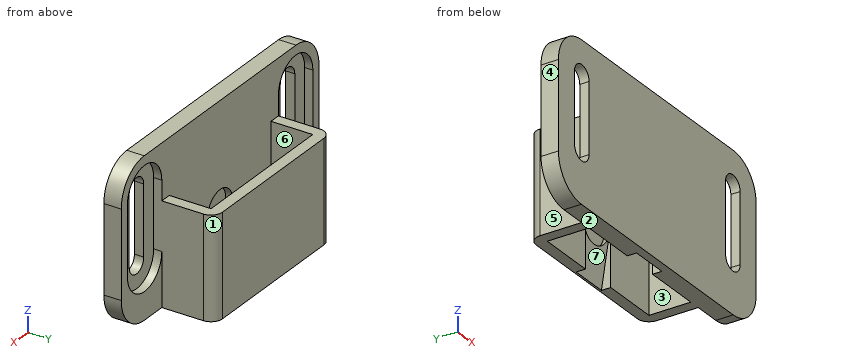
```python
from build123d import *

# Parameters (mm, degrees)
BOSS_EXTRUDE1_DEPTH = 3
CUT_EXTRUDE1_DEPTH  = 1.4
CUT_EXTRUDE2_DEPTH  = 3
BOSS_EXTRUDE2_DEPTH = 17.5
FILLET1_R           = 2
SKETCH8_R           = 3.3
CUT_EXTRUDE3_DEPTH  = 1.2
CUT_EXTRUDE4_START  = -1.2
SKETCH9_R           = 3.3
CUT_EXTRUDE4_DEPTH  = 1.2


with BuildPart() as part:
    # Sketch1 → Boss-Extrude1 (new body)
    with BuildSketch(Plane(origin=(0, 0, 0), x_dir=(1, 0, 0), z_dir=(0, 1, 0))):
        with BuildLine():
            Line((-19.85, -13.5), (19.85, -13.5))
            ThreePointArc((19.85, -13.5), (24.092640687, -11.742640687), (25.85, -7.5))
            Line((25.85, -7.5), (25.85, 7.5))
            ThreePointArc((25.85, 7.5), (24.092640687, 11.742640687), (19.85, 13.5))
            Line((19.85, 13.5), (-19.85, 13.5))
            ThreePointArc((-19.85, 13.5), (-24.092640687, 11.742640687), (-25.85, 7.5))
            Line((-25.85, 7.5), (-25.85, -7.5))
            ThreePointArc((-25.85, -7.5), (-24.092640687, -11.742640687), (-19.85, -13.5))
        make_face()
    extrude(amount=BOSS_EXTRUDE1_DEPTH)

    # Sketch2 → Cut-Extrude1 (cut)
    with BuildSketch(Plane(origin=(0, 3, 0), x_dir=(1, 0, 0), z_dir=(0, 1, 0))):
        with BuildLine():
            Line((-24.25, 4.3), (-24.25, -7.4))
            ThreePointArc((-24.25, -7.4), (-19.75, -11.9), (-15.25, -7.4))
            Line((-15.25, -7.4), (-15.25, 4.3))
            ThreePointArc((-15.25, 4.3), (-19.75, 8.8), (-24.25, 4.3))
        make_face()
        with BuildLine():
            Line((24.25, 4.3), (24.25, -7.4))
            ThreePointArc((24.25, -7.4), (19.75, -11.9), (15.25, -7.4))
            Line((15.25, -7.4), (15.25, 4.3))
            ThreePointArc((15.25, 4.3), (19.75, 8.8), (24.25, 4.3))
        make_face()
    extrude(amount=-CUT_EXTRUDE1_DEPTH, mode=Mode.SUBTRACT)

    # Sketch4 → Cut-Extrude2 (cut)
    with BuildSketch(Plane(origin=(0, 3, 0), x_dir=(1, 0, 0), z_dir=(0, 1, 0))):
        with BuildLine():
            Line((-17.85, 4.45), (-17.85, -7.55))
            ThreePointArc((-17.85, -7.55), (-19.75, -9.45), (-21.65, -7.55))
            Line((-21.65, -7.55), (-21.65, 4.45))
            ThreePointArc((-21.65, 4.45), (-19.75, 6.35), (-17.85, 4.45))
        make_face()
        with BuildLine():
            Line((17.85, 4.45), (17.85, -7.55))
            ThreePointArc((17.85, -7.55), (19.75, -9.45), (21.65, -7.55))
            Line((21.65, -7.55), (21.65, 4.45))
            ThreePointArc((21.65, 4.45), (19.75, 6.35), (17.85, 4.45))
        make_face()
    extrude(amount=-CUT_EXTRUDE2_DEPTH, mode=Mode.SUBTRACT)

    # Sketch5 → Boss-Extrude2 (add)
    with BuildSketch(Plane(origin=(0, 0, -13.5), x_dir=(-1, 0, 0), z_dir=(0, 0, -1))):
        Polygon((-13.3, 3), (-13.3, 10.2), (13.3, 10.2), (13.3, 3), (15.25, 3), (15.25, 12.15), (-15.25, 12.15), (-15.25, 3), align=None)
    extrude(amount=-BOSS_EXTRUDE2_DEPTH)

    # Fillet1
    fillet1_edges = [part.edges().sort_by_distance(p)[0] for p in [
        (15.25, 12.15, -4.75),
        (-15.25, 12.15, -4.75),
    ]]
    fillet(fillet1_edges, radius=FILLET1_R)

    # Sketch8 → Cut-Extrude3 (cut)
    with BuildSketch(Plane(origin=(0, 3, 0), x_dir=(1, 0, 0), z_dir=(0, 1, 0))):
        with Locations(Location((0, 4.4, 0), (0, 0, 270))):
            Circle(SKETCH8_R)
    extrude(amount=-CUT_EXTRUDE3_DEPTH, mode=Mode.SUBTRACT)

    # Sketch9 → Cut-Extrude4 (cut)
    with BuildSketch(Plane.XZ.offset(-10.2).offset(CUT_EXTRUDE4_START)):
        with Locations(Location((0, -4.4, 0), (0, 0, 90))):
            Circle(SKETCH9_R)
    extrude(amount=CUT_EXTRUDE4_DEPTH, mode=Mode.SUBTRACT)

    # Sketch11 → Cut-Loft4 section 0
    with BuildSketch(Plane(origin=(0, 0, -13.5), x_dir=(-1, 0, 0), z_dir=(0, 0, -1))):
        with BuildLine():
            Line((-3.3, 11.8), (3.3, 11.8))
            Line((3.3, 11.8), (3.3, 10.2))
            Line((3.3, 10.2), (-3.3, 10.2))
            Line((-3.3, 10.2), (-3.3, 11.8))
        make_face()
    # Sketch12 → Cut-Loft4 section 1
    with BuildSketch(Plane.XY.offset(-4.4)):
        with BuildLine():
            Line((-3.3, 10.2), (3.3, 10.2))
            Line((3.3, 10.2), (3.3, 10.4))
            Line((3.3, 10.4), (-3.3, 10.4))
            Line((-3.3, 10.4), (-3.3, 10.2))
        make_face()
    loft(mode=Mode.SUBTRACT)

    # Sketch11<110> → Cut-Loft7 section 0
    with BuildSketch(Plane(origin=(0, 0, -13.5), x_dir=(-1, 0, 0), z_dir=(0, 0, -1))):
        with BuildLine():
            Line((-3.3, 3), (3.3, 3))
            Line((3.3, 3), (3.3, 1.4))
            Line((3.3, 1.4), (-3.3, 1.4))
            Line((-3.3, 1.4), (-3.3, 3))
        make_face()
    # Sketch12<5> → Cut-Loft7 section 1
    with BuildSketch(Plane.XY.offset(-4.4)):
        with BuildLine():
            Line((-3.3, 3), (3.3, 3))
            Line((3.3, 3), (3.3, 2.8))
            Line((3.3, 2.8), (-3.3, 2.8))
            Line((-3.3, 2.8), (-3.3, 3))
        make_face()
    loft(mode=Mode.SUBTRACT)


solid = part.part
```
Geometry: final body of the model. Coordinates: model frame, mm. Face numbers are marked on the shaded views. A direction names the side the tool comes from. Coordinates: 2 decimals unless noted, no trailing zeros. Order: outer loops, then holes, each group sorted by start corner. A loop starts at its lowest first (then second) coordinate and runs counter-clockwise, first axis right, second up.
Item 1: Section query C-C (x = 14). Output: boundary loops of the cut face in (y, z).
Answer:
outline: (0, -13.5) - (12, -13.5) - (12, 4) - (3, 4) - (3, 13.5) - (0, 13.5) - close
Item 2: Contact query for flat-ended pins moving along their axis: P1, Ø4.5, axis at y = 7.5, z = -2, coming from the -X side; P2, Ø6, axis at x = 19, z = -7, coming from the +Y side; P3, Ø1.5, axis at x = 18, z = -7.5, coming from the +Y side. Output: stop coordinate, or through.
Answer:
P1: stops at x = -15.25
P2: stops at y = 3
P3: stops at y = 1.6
Item 3: Material intervals for line 1 along X through (y, z) = (2, 2); line 2 along X through (y, z) = (2.3, -4.4); line 3 along Y through (x, z) = (-7, 0.75), sorted ascending.
Answer:
line 1: x = -25.85 to -24.25, -15.25 to 15.25, 24.25 to 25.85
line 2: x = -25.85 to -24.25, -15.25 to -3.3, 3.3 to 15.25, 24.25 to 25.85
line 3: y = 0 to 3, 10.2 to 12.15
Item 4: Access query for the marked faces 5, 6 and 7. Directions: +Z, -Z, +X, -X, +Y, -Y. A direction counts if a zero-diameter tool reaches every point of the face in a straight line with its end or side. Return the directions, or none.
Answer:
face 5: +Y
face 6: +Z, -Z
face 7: -Z
Item 5: Section query B-B (x = -1). Output: boundary loops of the cut face in (y, z), then the cut area to 3 significant figures.
Answer:
outline: (0, -13.5) - (1.4, -13.5) - (2.32, -7.54) - (1.8, -7.54) - (1.8, -1.26) - (3, -1.26) - (3, 13.5) - (0, 13.5) - close; (10.2, -1.26) - (11.4, -1.26) - (11.4, -7.54) - (10.88, -7.54) - (11.8, -13.5) - (12.15, -13.5) - (12.15, 4) - (10.2, 4) - close
area: 86.4 mm2
Item 6: Draft query along X for the marked faces 1, 2, 3 and 4. Return one class per face: released by +X, released by -X, zero draft, split by the parting line, or undercut.
Answer:
face 1: released by +X
face 2: zero draft
face 3: undercut
face 4: released by -X
Item 7: Section query A-A (y = 4.5). Output: boundary loops of the cut face in (x, z), then the cut area to 4 significant figures.
Answer:
outline: (-15.25, -13.5) - (-13.3, -13.5) - (-13.3, 4) - (-15.25, 4) - close; (13.3, -13.5) - (15.25, -13.5) - (15.25, 4) - (13.3, 4) - close
area: 68.25 mm2
